Design review of the part built by this model. Coordinates are the model's own, in mm. Face numbers are marked on the shaded views. Coordinates: 2 decimals unless noted, no trailing zeros. Loops run counter-clockwise (first coordinate to the right, second up) from the corner with the lowest first, then second, coordinate; pieces in that order, holes last. Notation, with made-up numbers: (49.25, 8) -> (55.25, 8) arc R12 cw to (55.25, 22) -> close; hole circle Ø4 at (-28, 31.5). An arc over 180 degrees is marked (long way). Use a Markdown table: item, result. Add a question column.
Q1. Take a section at B-B on y = 0. Write out the cut boundary in (x, z), plus the area to 3 significant figures.
Q2. Draft analysis for pull direction Y (two halves, no side actions). For the marked faces 1 and 2, state which applies: pulls with the +Y half, pulls with the -Y half, needs draft (parallel to the pull), parting line crosses it, or undercut.
Q3. For probe 1 along X at (y, z) = (-0.25, 58); probe 2 along Y at (x, z) = (2, 34); probe 3 along Z at (x, y) = (13, -0.5), list the stretches that pass through material, from the lowest coordinate up.
Q4. Take a section at D-D on z = 7.5. Write out the cut boundary in (x, y).
Q5. Clearance check with flat-ended pins moving along their axes: pin 1 Ø10 at (x, z) = (6.5, 23.5) entering from +Y; pin 2 Ø2 at (y, z) = (1, 58.5) entering from +X; pin 3 Ø1 at (x, y) = (4, 0.5) entering from +Z. State where each tip first meets the part, or that it passes through.
Q6. Take a section at A-A on z = 62. Write out the cut boundary in (x, y).
Q7. Take a section at C-C on x = -5. Write out the cut boundary in (y, z).
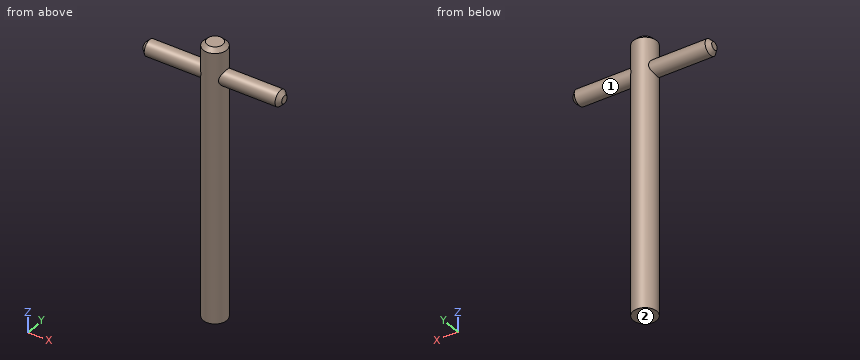
Autodesk Inventor part; units mm, degrees
ref_plane "YZ Plane" through (0, 0, 0) normal (1, 0, 0) x (0, 1, 0)
ref_plane "XZ Plane" through (0, 0, 0) normal (0, 1, 0) x (-1, 0, 0)
ref_plane "XY Plane" through (0, 0, 0) normal (0, 0, 1) x (1, 0, 0)
sketch "Sketch1" plane through (0, 0, 0) normal (0, 0, 1) x (1, 0, 0)
  circle A0 centre (0, 0) radius 3
  dimension "d0" = 6
extrude "Extrusion1" add sketch "Sketch1" along normal blind 70
thread "Thread1"
chamfer "Chamfer1" distance 1 angle 45 1 edges at (-3, 0, 70)
sketch "Sketch2" plane through (0, 0, 0) normal (1, 0, 0) x (0, 1, 0)
  line L0 (-2, 70) -> (2, 70) construction
  line L1 (0, 70) -> (0, 62) construction
  circle A0 centre (0, 62) radius 2
  point P0 (0, 0)
  dimension "d8" = 8
  dimension "d9" = 4
extrude "Extrusion2" add sketch "Sketch2" along normal mid plane 35
chamfer "Chamfer2" distance 1 angle 45 2 edges at (17.5, -2, 62) (-17.5, -2, 62)
properties part number "screw"
Answer list:
| question | item | result |
|---|---|---|
| 1 | outline | (-17.5, 61) -> (-16.5, 60) -> (-3, 60) -> (-3, 0) -> (3, 0) -> (3, 60) -> (16.5, 60) -> (17.5, 61) -> (17.5, 63) -> (16.5, 64) -> (3, 64) -> (3, 69) -> (2, 70) -> (-2, 70) -> (-3, 69) -> (-3, 64) -> (-16.5, 64) -> (-17.5, 63) -> close |
| 1 | area | 533 mm² |
| 2 | face 1 | parting line crosses it |
| 2 | face 2 | needs draft |
| 3 | probe 1 | -2.99 to 2.99 |
| 3 | probe 2 | -2.24 to 2.24 |
| 3 | probe 3 | 60.06 to 63.94 |
| 4 | outline | circle Ø6 at (0, 0) |
| 5 | pin 1 | y = 2.6 |
| 5 | pin 2 | x = 3 |
| 5 | pin 3 | z = 64 |
| 6 | outline | (-17.5, -1) -> (-16.5, -2) -> (-2.24, -2) arc R3 ccw to (2.24, -2) -> (16.5, -2) -> (17.5, -1) -> (17.5, 1) -> (16.5, 2) -> (2.24, 2) arc R3 ccw to (-2.24, 2) -> (-16.5, 2) -> (-17.5, 1) -> close |
| 7 | outline | circle Ø4 at (0, 62) |
